Build history of the part. All positions in model axes, mm. Round coordinates to 2 decimals unless told otherwise and drop trailing zeros. Loops run counter-clockwise (first coordinate to the right, second up) from the corner with the lowest first, then second, coordinate; pieces in that order, holes last.
Autodesk Inventor part; units mm, degrees
ref_plane "YZ Plane" through (0, 0, 0) normal (1, 0, 0) x (0, 1, 0)
ref_plane "XZ Plane" through (0, 0, 0) normal (0, 1, 0) x (-1, 0, 0)
ref_plane "XY Plane" through (0, 0, 0) normal (0, 0, 1) x (1, 0, 0)
sketch "Sketch1" plane through (0, 0, 0) normal (0, 1, 0) x (-1, 0, 0)
  line L0 (0, 0) -> (0, 50.8)
  line L1 (0, 50.8) -> (50.8, 50.8)
  line L2 (50.8, 50.8) -> (50.8, 0)
  line L3 (50.8, 0) -> (0, 0)
  circle A0 centre (6.35, 40.4012) radius 2.8956
  circle A1 centre (6.35, 10.4013) radius 2.8956
  circle A2 centre (39.9999, 25.4) radius 3.4925
  dimension "d0" = 50.8
  dimension "d1" = 50.8
  dimension "d2" = 5.7912
  dimension "d3" = 5.7912
  dimension "d4" = 29.9999
  dimension "d5" = 10.4013
  dimension "d6" = 6.35
  dimension "d7" = 6.35
  dimension "d8" = 6.985
  dimension "d9" = 39.9999
  dimension "d10" = 25.4
extrude "Extrusion1" add sketch "Sketch1" along normal blind 25.4
properties part number "SpoutHolder"
(1) Probe line 1 (Z direction, x = -6.35, y = 17); line 2 (Z direction, x = -8.5, y = 9.25); line 3 (X direction, y = 13.5, z = 28.5). List the from-to ranges inside material, lowest first.
Responses:
line 1: z = 0 to 7.51, 13.3 to 37.51, 43.3 to 50.8
line 2: z = 0 to 8.46, 12.34 to 38.46, 42.34 to 50.8
line 3: x = -50.8 to -41.61, -38.39 to 0
(2) Slice it at D-D on z = 12. List the corners of the cut face in (x, y), plus the area to 3 significant figures.
Responses:
outline: (-50.8, 0) - (-8.76, 0) - (-8.76, 25.4) - (-50.8, 25.4) - close; (-3.94, 0) - (0, 0) - (0, 25.4) - (-3.94, 25.4) - close
area: 1,170 mm2
(3) Slice it at B-B on z = 25.4. List the corners of the cut face in (x, y), plus the area to 3 significant figures.
Responses:
outline: (-50.8, 0) - (-43.49, 0) - (-43.49, 25.4) - (-50.8, 25.4) - close; (-36.51, 0) - (0, 0) - (0, 25.4) - (-36.51, 25.4) - close
area: 1,110 mm2
(4) Pin check, flat tip, straight feed: P1, Ø1.5, axis at x = -26.5, y = 20.5, coming from the -Z side. Stop position of the tip, or through.
Responses:
P1: stops at z = 0
(5) Slice it at C-C on y = 14. Count the separate pieces of the cut face and the enclosed holes in it, plus the area to 3 significant figures.
Responses:
separate pieces: 1
enclosed holes: 3
area: 2,490 mm2
(6) Pull direction Z, two halves, no side cores. Call faces 1 (the face through (-9.025, 12.522, 11.51)), 2 (the face through (-26, 13, 0)), 3 (the face through (-25, 0, 26)): +Z half, -Z half, draft (parallel to the pull), parting line (faces both ways), or undercut.
Responses:
face 1: undercut
face 2: -Z half
face 3: draft
(7) Slice it at A-A on x = -6.35. List the corners of the cut face in (y, z).
Responses:
outline: (0, 0) - (25.4, 0) - (25.4, 7.51) - (0, 7.51) - close; (0, 13.3) - (25.4, 13.3) - (25.4, 37.51) - (0, 37.51) - close; (0, 43.3) - (25.4, 43.3) - (25.4, 50.8) - (0, 50.8) - close
